from build123d import *

# Parameters (mm, degrees)
F0_R     = 14
F0_R_2   = 8
F1_DEPTH = 31
F2_R     = 14
F2_R_2   = 8
F3_DEPTH = 10
F5_D     = 5


with BuildPart() as f1:
    # F0 (on Top) → F1 (new body)
    with BuildSketch(Plane.XY):
        with Locations((-24.742087, 7.847304)):
            Circle(F0_R)
        with Locations((-24.742087, 7.847304)):
            Circle(F0_R_2, mode=Mode.SUBTRACT)
    extrude(amount=F1_DEPTH)

    # F2 (on face) → F3 (join)
    with BuildSketch(Plane.XY.offset(31)):
        with BuildLine():
            Line((-4.742087, -5.419196), (-4.742087, 21.113803))
            ThreePointArc((-4.742087, 21.113803), (-24.742087, 31.847304), (-44.742087, 21.113803))
            Line((-44.742087, 21.113803), (-44.742087, -5.419196))
            ThreePointArc((-44.742087, -5.419196), (-24.742087, -16.152696), (-4.742087, -5.419196))
        make_face()
        with Locations((-24.742087, 7.847304)):
            Circle(F2_R, mode=Mode.SUBTRACT)
        with Locations((-24.742087, 7.847304)):
            Circle(F2_R)
        with Locations((-24.742087, 7.847304)):
            Circle(F2_R_2, mode=Mode.SUBTRACT)
    extrude(amount=F3_DEPTH)

    # F5 (through all)
    with Locations(Plane.XY.offset(41)):
        with Locations((-38.177116, 21.282332), (-24.742087, 26.847304), (-11.307059, 21.282332), (-11.307059, -5.587725), (-24.742087, -11.152696), (-38.177116, -5.587725)):
            Hole(F5_D / 2)


solid = f1.part
Can you work these out from the model? Positions are in its coordinate system, mm. A direction names the side the tool comes from. Round coordinates to 2 decimals unless told otherwise and drop trailing zeros. Write each loop counter-clockwise with the first axis right and the second up, starting at its lowest first coordinate (ties: lowest second). Pieces come first, ordered by that corner, then holes. Notation, with made-up numbers: M -36.75,55 L 7.25,55 A26 cw 7.25,72 Z; hole C 27,-16 d9. An arc over 180 degrees is marked long. Use a Markdown table: item, result.
Item 1: If I drill on line 1 along X through (y, z) = (8, 27.5); line 2 along Z through (x, y) = (-12.5, 0.5); line 3 along X through (y, z) = (-6, 39.5), over which ranges is the centre line in solid material (lowest first)? Write a range as [from, to].
Found:
| item | result |
|---|---|
| line 1 | x = [-38.74, -32.74], [-16.74, -10.74] |
| line 2 | z = [31, 41] |
| line 3 | x = [-44.34, -40.64], [-35.71, -13.77], [-8.84, -5.14] |
Item 2: We'd pull the mould along Y, two halves only. Please class faces 1 (the face through (-44.742, 8, 36)), 2 (the face through (-24.411, 31.845, 35.93)), 3 (the face through (-35.68, -5.48, 35.93)): released by +Y, released by -Y, zero draft, split by the parting line, or undercut.
Found:
| item | result |
|---|---|
| face 1 | zero draft |
| face 2 | released by +Y |
| face 3 | undercut |
Item 3: I want a section at B-B (z = 36). List the corners of the cut face in (x, y) for me.
Found:
| item | result |
|---|---|
| outline | M -44.74,-5.42 A24 ccw -4.74,-5.42 L -4.74,21.11 A24 ccw -44.74,21.11 Z; hole C -38.18,-5.59 d5; hole C -38.18,21.28 d5; hole C -24.74,7.85 d16; hole C -24.74,-11.15 d5; hole C -24.74,26.85 d5; hole C -11.31,-5.59 d5; hole C -11.31,21.28 d5 |
Item 4: Which directions (+Z, -Z, +X, -X, +Y, -Y) give clear straight access to the entire face, cutting with the end or side of a thin tool? Please do faces 4 (the face through (-34, 19, 31)), 5 (the face through (-16, 8, 41)).
Found:
| item | result |
|---|---|
| face 4 | -Z |
| face 5 | +Z, +X, -X, +Y, -Y |
Item 5: I want a section at C-C (x = -26.5). List the corners of the cut face in (y, z) for me.
Found:
| item | result |
|---|---|
| outline | M -16.09,31 L -12.93,31 L -12.93,41 L -16.09,41 Z; M -9.38,31 L -6.04,31 L -6.04,0 L 0.04,0 L 0.04,41 L -9.38,41 Z; M 15.65,0 L 21.74,0 L 21.74,31 L 25.07,31 L 25.07,41 L 15.65,41 Z; M 28.62,31 L 31.78,31 L 31.78,41 L 28.62,41 Z |
Item 6: For pin 1 Ø3 at (x, y) = (-38.18, -5.59) entering from +Z; pin 2 Ø4 at (y, z) = (1.5, 18) entering from -X; pin 3 Ø6 at (x, z) = (-38, 31) entering from -Y; pin 4 Ø3 at (y, z) = (-11, 34) entering from +X, each with a flat end and sliding along its axis, tell me the tip position at first contact or that it passes through.
Found:
| item | result |
|---|---|
| pin 1 | passes through |
| pin 2 | stops at x = -38.05 |
| pin 3 | stops at y = -13.85 |
| pin 4 | stops at x = -8.16 |
Item 7: I want a section at D-D (y = 22.5). List the corners of the cut face in (x, z) for me.
Found:
| item | result |
|---|---|
| outline | M -43.75,31 L -40.36,31 L -40.36,41 L -43.75,41 Z; M -35.99,31 L -13.49,31 L -13.49,41 L -35.99,41 Z; M -9.12,31 L -5.73,31 L -5.73,41 L -9.12,41 Z |
Item 8: I want a section at A-A (x = -18.5). List the corners of the cut face in (y, z) for me, and give its area (3 significant figures).
Found:
| item | result |
|---|---|
| outline | M -15.33,31 L -4.68,31 L -4.68,0 L 2.84,0 L 2.84,41 L -15.33,41 Z; M 12.85,0 L 20.38,0 L 20.38,31 L 31.02,31 L 31.02,41 L 12.85,41 Z |
| area | 830 mm2 |
